```python
from build123d import *

# Parameters (mm, degrees)
SKETCH1_W                 = 25.4
SKETCH1_H                 = 7.62
BOSS_EXTRUDE1_DEPTH       = 3.81
TAP_DRILL_FOR_6_32_TAP1_D = 2.7051
TAP_DRILL_FOR_6_32_TAP2_D = 2.7051


with BuildPart() as part:
    # Sketch1 → Boss-Extrude1 (new, symmetric)
    with BuildSketch(Plane(origin=(0, 0, 0), x_dir=(1, 0, 0), z_dir=(0, 1, 0))):
        Rectangle(SKETCH1_W, SKETCH1_H)
    extrude(amount=BOSS_EXTRUDE1_DEPTH, both=True)

    # Tap Drill for #6-32 Tap1 (through all)
    with Locations(Plane(origin=(0, 3.81, 0), x_dir=(1, 0, 0), z_dir=(0, 1, 0))):
        with Locations((-8.89, 0), (3.81, 0)):
            Hole(TAP_DRILL_FOR_6_32_TAP1_D / 2)

    # Tap Drill for #6-32 Tap2 (through all)
    with Locations(Plane.XY.offset(3.81)):
        with Locations((-3.81, 0), (8.89, 0)):
            Hole(TAP_DRILL_FOR_6_32_TAP2_D / 2)


solid = part.part
```
The listing builds one solid part. Answer for the finished solid, in the listing's coordinates (mm). Round coordinates to 2 decimals unless told otherwise and drop trailing zeros. Loops run counter-clockwise (first coordinate to the right, second up) from the corner with the lowest first, then second, coordinate; pieces in that order, holes last.
Q1. Section A-A, the plane y = 0 is taken. Determine the outline of the cut face in (x, z), then the cut area to 3 significant figures.
Q2. For a pull along Y with two mould halves and no side action, classify faces 1 (the face through (-5.06, -0.52, -0.05)), 2 (the face through (0, 0, 3.81)), 3 (the face through (0, -3.81, 0)) as released by +Y, released by -Y, zero draft, split by the parting line, or undercut.
Q3. Section D-D, the plane z = 2.75 is taken. Determine the outline of the cut face in (x, y), then the cut area to 3 significant figures.
Q4. Section B-B, the plane z = 0.25 is taken. Determine the outline of the cut face in (x, y).
Q5. Section C-C, the plane x = -3.81 is taken. Determine the outline of the cut face in (y, z).
Q6. Find the intervals of material crossed by line 1 (Z direction, x = 3.81, y = -1.5), in increasing order.
Completed:
1. outline: (-12.7, -3.81) - (-5.16, -3.81) - (-5.16, 3.81) - (-12.7, 3.81) - close; (-2.46, -3.81) - (7.54, -3.81) - (7.54, 3.81) - (-2.46, 3.81) - close; (10.24, -3.81) - (12.7, -3.81) - (12.7, 3.81) - (10.24, 3.81) - close; hole circle Ø2.71 at (-8.89, 0); hole circle Ø2.71 at (3.81, 0)
1. area: 141 mm2
2. face 1: undercut
2. face 2: zero draft
2. face 3: released by -Y
3. outline: (-12.7, -3.81) - (12.7, -3.81) - (12.7, 3.81) - (-12.7, 3.81) - close; hole circle Ø2.71 at (-3.81, 0); hole circle Ø2.71 at (8.89, 0)
3. area: 182 mm2
4. outline: (-12.7, -3.81) - (-10.22, -3.81) - (-10.22, 3.81) - (-12.7, 3.81) - close; (-7.56, -3.81) - (2.48, -3.81) - (2.48, 3.81) - (-7.56, 3.81) - close; (5.14, -3.81) - (12.7, -3.81) - (12.7, 3.81) - (5.14, 3.81) - close; hole circle Ø2.71 at (-3.81, 0); hole circle Ø2.71 at (8.89, 0)
5. outline: (-3.81, -3.81) - (-1.35, -3.81) - (-1.35, 3.81) - (-3.81, 3.81) - close; (1.35, -3.81) - (3.81, -3.81) - (3.81, 3.81) - (1.35, 3.81) - close
6. line 1: z = -3.81 to -1.35, 1.35 to 3.81
